Build history of the part. All positions in model axes, mm. Give positions to 0.01 mm unless a question says otherwise; leave off trailing zeros. Loops run counter-clockwise (first coordinate to the right, second up) from the corner with the lowest first, then second, coordinate; pieces in that order, holes last.
1) Wall check: line 1 (X direction, y = 226.5, z = -4); line 2 (X direction, y = 280.5, z = -8.25); line 3 (Z direction, x = 12, y = 199). Give the ranges that are in metal, low to high.
2) Band-saw the part on B-B on y = 293.5. List the corners of the cut face in (x, z).
3) Band-saw the part on A-A on y = 123.5. List the corners of the cut face in (x, z), then the cut area to 3 significant figures.
4) Flat gauge pins, fed straight in: P1, Ø1.5, axis at y = 292.5, z = -4, coming from the +X side; P2, Ø4, axis at y = 374.5, z = -9.5, coming from the -X side; P3, Ø3, axis at y = 348.5, z = -10, coming from the +X side. Where does each tip first touch, or does it go through?
Autodesk Inventor part; units mm, degrees
ref_plane "Work Plane1" through (15, 0, 0) normal (1, 0, 0) x (0, 1, 0)
ref_plane "Work Plane2" through (0, 0, 15) normal (0, 0, 1) x (1, 0, 0)
ref_plane "XZ Plane" through (0, 0, 0) normal (0, 1, 0) x (-1, 0, 0)
sketch "Sketch1" plane through (0, 0, 0) normal (0, 1, 0) x (-1, 0, 0)
  circle A0 centre (0, 0) radius 15
  dimension "d0" = 30
extrude "Extrusion1" add sketch "Sketch1" along normal blind 500
ref_plane "Work Plane1" through (15, 0, 0) normal (1, 0, 0) x (0, 1, 0)
sketch "Sketch2" plane through (15, 0, 0) normal (1, 0, 0) x (0, 1, 0)
  line L0 (50, 4.712) -> (50, -4.713)
  line L1 (450, 0) -> (50, -4.713)
  line L2 (50, 4.712) -> (450, 0)
  point P0 (0, 0)
  dimension "d4" = 9.425
extrude "Extrusion2" cut sketch "Sketch2" against normal blind 500
ref_plane "Work Plane2" through (0, 0, 15) normal (0, 0, 1) x (1, 0, 0)
sketch "Sketch3" plane through (0, 0, 15) normal (0, 0, 1) x (1, 0, 0)
  line L0 (4.712, 50) -> (-4.713, 50)
  line L1 (0, 450) -> (4.712, 50)
  line L2 (0, 450) -> (-4.713, 50)
  point P0 (0, 0)
  dimension "d8" = 9.425
extrude "Extrusion3" cut sketch "Sketch3" against normal blind 500
sketch "Sketch4" plane through (0, 500, 0) normal (0, 1, 0) x (1, 0, 0)
  circle A0 centre (0, 0) radius 10
  dimension "d11" = 20
extrude "Extrusion4" cut sketch "Sketch4" against normal blind 500
sketch "Sketch5" plane through (0, 500, 0) normal (0, 1, 0) x (1, 0, 0)
  circle A0 centre (0, 0) radius 15
extrude "Extrusion5" cut sketch "Sketch5" against normal blind 10
sketch "Sketch6" plane through (0, 0, 0) normal (0, -1, 0) x (1, 0, 0)
  circle A0 centre (0, 0) radius 15
extrude "Extrusion6" cut sketch "Sketch6" against normal blind 10
sketch "Sketch7" plane through (0, 0, 0) normal (0, 0, 1) x (1, 0, 0)
  point P0 (0, 0)
sketch "Sketch8" plane through (0, 10, 0) normal (0, -1, 0) x (1, 0, 0)
  circle A0 centre (0, 0) radius 15
extrude "Extrusion7" cut sketch "Sketch8" against normal blind 10
sketch "Sketch9" plane through (0, 490, 0) normal (0, 1, 0) x (1, 0, 0)
  circle A0 centre (0, 0) radius 10
  circle A1 centre (0, 0) radius 15
extrude "Extrusion8" cut sketch "Sketch9" against normal blind 10
sketch "Sketch10" plane through (0, 20, 0) normal (0, -1, 0) x (1, 0, 0)
  arc A0 (14.2404, -4.713) -> (14.2407, 4.712) centre (0, 0) ccw
  circle A1 centre (0, 0) radius 15
extrude "Extrusion9" cut sketch "Sketch10" against normal blind 15
sketch "Sketch11" plane through (0, 480, 0) normal (0, 1, 0) x (1, 0, 0)
  arc A0 (14.2407, -4.712) -> (15, 0) centre (0, 0) ccw
  circle A1 centre (0, 0) radius 15
extrude "Extrusion10" cut sketch "Sketch11" against normal blind 15
properties part number "steam pipe"
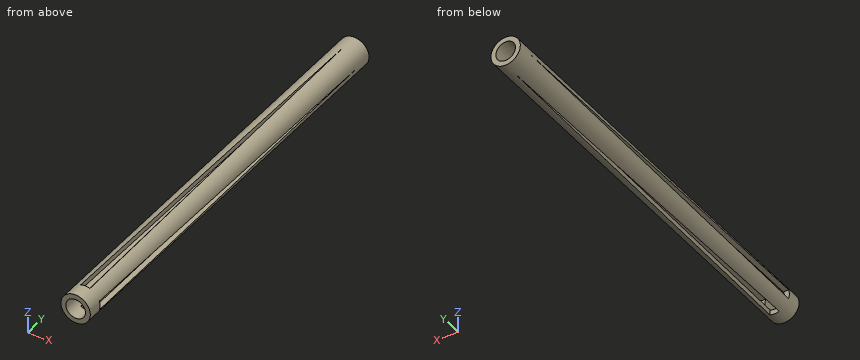
Findings below:
1. line 1: x = -14.46 to -9.17, 9.17 to 14.46
1. line 2: x = -12.53 to -5.65, 5.65 to 12.53
1. line 3: z = -9 to -2.96, 2.96 to 9
2. outline: (-14.89, -1.84) arc R15 ccw to (-1.84, -14.89) - (-1.84, -9.83) arc R10 cw to (-9.83, -1.84) - close; (-14.89, 1.84) - (-9.83, 1.84) arc R10 cw to (-1.84, 9.83) - (-1.84, 14.89) arc R15 ccw to start; (1.84, -14.89) arc R15 ccw to (14.89, -1.84) - (9.83, -1.84) arc R10 cw to (1.84, -9.83) - close; (1.84, 9.83) arc R10 cw to (9.83, 1.84) - (14.89, 1.84) arc R15 ccw to (1.84, 14.89) - close
3. outline: (-14.5, -3.85) arc R15 ccw to (-3.85, -14.5) - (-3.85, -9.23) arc R10 cw to (-9.23, -3.85) - close; (-14.5, 3.85) - (-9.23, 3.85) arc R10 cw to (-3.85, 9.23) - (-3.85, 14.5) arc R15 ccw to start; (3.85, -14.5) arc R15 ccw to (14.5, -3.85) - (9.23, -3.85) arc R10 cw to (3.85, -9.23) - close; (3.85, 9.23) arc R10 cw to (9.23, 3.85) - (14.5, 3.85) arc R15 ccw to (3.85, 14.5) - close
3. area: 236 mm2
4. P1: stops at x = 14.64
4. P2: stops at x = -12.99
4. P3: stops at x = 12.36
